Source: CAD feature listing. Evaluate the final solid. Frame: model axes, mm. A direction names the side the tool comes from. Coordinates: 2 decimals unless noted, no trailing zeros. Loops run counter-clockwise (first coordinate to the right, second up) from the corner with the lowest first, then second, coordinate; pieces in that order, holes last. Notation, with made-up numbers: (22.5, 73) - (36.5, 73) arc R16 ccw to (36.5, 95) - close; hole circle Ø10 at (63, 80). An arc over 180 degrees is marked (long way). Use one line per item in the form item = value. Start each with the question number.
from build123d import *

# Parameters (mm, degrees)
BOSS_EXTRUDE1_DEPTH = 50
SKETCH2_R           = 30
CUT_EXTRUDE1_DEPTH  = 50


with BuildPart() as part:
    # Sketch1 → Boss-Extrude1 (new body)
    with BuildSketch(Plane(origin=(0, 0, 0), x_dir=(1, 0, 0), z_dir=(0, 1, 0))):
        with BuildLine():
            Line((-20, 50), (20, 50))
            Line((20, 50), (20, 34.818623064))
            ThreePointArc((20, 34.818623064), (40.154606831, 0.088803456), (20, -34.641016151))
            Line((20, -34.641016151), (20, -50))
            Line((20, -50), (-20, -50))
            Line((-20, -50), (-20, -34.641016151))
            ThreePointArc((-20, -34.641016151), (-40, 0), (-20, 34.641016151))
            Line((-20, 34.641016151), (-20, 50))
        make_face()
    extrude(amount=BOSS_EXTRUDE1_DEPTH)

    # Sketch2 → Cut-Extrude1 (cut)
    with BuildSketch(Plane(origin=(0, 50, 0), x_dir=(1, 0, 0), z_dir=(0, 1, 0))):
        Circle(SKETCH2_R)
    extrude(amount=-CUT_EXTRUDE1_DEPTH, mode=Mode.SUBTRACT)


solid = part.part
(1) Access query for faces 5 (the face through (-20, 25, 42)), 6 (the face through (0, 25, 50)), 7 (the face through (20, 25, 42)), 8 (the face through (20, 25, -43)), 9 (the face through (1, 0, -34)). Directions: +Z, -Z, +X, -X, +Y, -Y. A direction counts if a zero-diameter tool reaches every point of the face in a straight line with its end or side. Return the directions, or none.
(2) Cut plane B-B, the plane z = 0. Output: boundary loops of the cut face in (x, y), plus the area to 3 significant figures.
(3) Material intervals for line 1 (Z direction, x = 0, y = 19); line 2 (X direction, y = 38.5, z = 7); line 3 (X direction, y = 41.5, z = -46), sorted ascending.
(4) Cut plane A-A, the plane x = 0. Output: boundary loops of the cut face in (y, z).
(5) Mould query, pull axis Z, two halves, no side actions, for faces 1 (the face through (0, 25, -50)), 2 (the face through (-39.996, 24.65, 0.586)), 3 (the face through (-29.97, 25.35, -1.32)), 4 (the face through (-20, 25, -42)). Classes: +Z half, -Z half, draft (parallel to the pull), parting line (faces both ways), or undercut.
(6) Cut plane C-C, the plane y = 11. Output: boundary loops of the cut face in (x, z), plus the area to 3 significant figures.
(7) Contact query for flat-ended pins moving along their axis: pin 1 (7.5 mm diameter, centred on y = 13, z = -42, fed in from +X); pin 2 (12.5 mm diameter, centred on y = 30.5, z = -39, fed in from -X); pin 3 (3 mm diameter, centred on x = -23, y = 28, fed in from +Z). Output: stop coordinate, or through.
(8) Cut plane D-D, the plane x = -31.5. Output: boundary loops of the cut face in (y, z).
Recorded:
q1.face_5 = +Z, -X, +Y, -Y
q1.face_6 = +Z, +X, -X, +Y, -Y
q1.face_7 = +Z, +X, +Y, -Y
q1.face_8 = -Z, +X, +Y, -Y
q1.face_9 = +Z, -Z, +X, -X, -Y
q2.outline = (-40, 0) - (-30, 0) - (-30, 50) - (-40, 50) - close; (30, 0) - (40.15, 0) - (40.15, 50) - (30, 50) - close
q2.area = 1,010 mm²
q3.line_1 = -50 to -30, 30 to 50
q3.line_2 = -39.38 to -29.17, 29.17 to 39.52
q3.line_3 = -20 to 20
q4.outline = (0, -50) - (50, -50) - (50, -30) - (0, -30) - close; (0, 30) - (50, 30) - (50, 50) - (0, 50) - close
q5.face_1 = -Z half
q5.face_2 = parting line
q5.face_3 = undercut
q5.face_4 = draft
q6.outline = (-20, -50) - (20, -50) - (20, -34.82) arc R40 ccw to (20, 34.64) - (20, 50) - (-20, 50) - (-20, 34.64) arc R40 ccw to (-20, -34.64) - close; hole circle Ø60 at (0, 0)
q6.area = 3,150 mm²
q7.pin_1 = 20
q7.pin_2 = -22.97
q7.pin_3 = 33.73
q8.outline = (0, -24.65) - (50, -24.65) - (50, 24.65) - (0, 24.65) - close
